Model file for the job. Use its own axes, mm. A direction names the side the tool comes from. Give positions to 0.01 mm unless a question says otherwise; leave off trailing zeros. Write each loop counter-clockwise with the first axis right and the second up, starting at its lowest first coordinate (ties: lowest second). Pieces come first, ordered by that corner, then holes. Notation, with made-up numbers: (51.25, -0.5) - (88.25, -0.5) arc R11 ccw to (88.25, 9.5) - close; hole circle Ø8 at (57, -17.5). An arc over 180 degrees is marked (long way). Use CSV: the item, a comma, the result in double quotes.
from build123d import *

# Parameters (mm, degrees)
BOSS_EXTRUDE1_DEPTH     = 1.5
BOSS_EXTRUDE2_DEPTH     = 280
SKETCH4_W               = 400
SKETCH4_H               = 42.385541564
BOSS_EXTRUDE3_DEPTH     = 2
CUT_EXTRUDE1_DEPTH      = 609.61485268
CUT_EXTRUDE1_DEPTH_BACK = 609.61485268
SKETCH8_R               = 4.39
SKETCH8_R_2             = 2.39
BOSS_EXTRUDE5_DEPTH     = 15
SKETCH10_R              = 3
CUT_EXTRUDE2_DEPTH      = 2
SKETCH15_W              = 15
SKETCH15_H              = 1.5
BOSS_EXTRUDE6_DEPTH     = 15
BOSS_EXTRUDE7_DEPTH     = 1.5
BOSS_EXTRUDE8_DEPTH     = 1.5
SKETCH20_R              = 2.415919743
SKETCH20_R_2            = 2
CUT_EXTRUDE5_DEPTH      = 1.5
SKETCH5_R               = 2
SKETCH5_R_2             = 10
CUT_EXTRUDE7_DEPTH      = 2
SKETCH21_W              = 300
SKETCH21_H              = 1.5
BOSS_EXTRUDE9_DEPTH     = 10
SKETCH22_W              = 300
SKETCH22_H              = 1.5
BOSS_EXTRUDE10_DEPTH    = 10
BOSS_EXTRUDE11_DEPTH    = 0.75
BOSS_EXTRUDE12_DEPTH    = 0.75
BOSS_EXTRUDE13_DEPTH    = 0.75
BOSS_EXTRUDE14_DEPTH    = 0.75
SKETCH27_W              = 200
SKETCH27_H              = 1.5
BOSS_EXTRUDE15_DEPTH    = 10
BOSS_EXTRUDE16_DEPTH    = 0.75
BOSS_EXTRUDE17_DEPTH    = 0.75
SKETCH30_R              = 24
SKETCH30_R_2            = 1.5
CUT_EXTRUDE8_DEPTH      = 2
SKETCH33_R              = 2
CUT_EXTRUDE9_DEPTH      = 2
SKETCH42_W              = 396
SKETCH42_H              = 39.39
CUT_EXTRUDE13_DEPTH     = 40


with BuildPart() as part:
    # Sketch1 → Boss-Extrude1 (new body)
    with BuildSketch(Plane(origin=(0, 0, 0), x_dir=(1, 0, 0), z_dir=(0, 1, 0))):
        Polygon((-200, 237.826300096), (200, 237.826300096), (200, -292.173699904), (150, -292.173699904), (150, -362.173699904), (-200, -362.173699904), align=None)
    extrude(amount=BOSS_EXTRUDE1_DEPTH)

    # Sketch2 → Boss-Extrude2 (add)
    with BuildSketch(Plane(origin=(0, 1.5, 0), x_dir=(1, 0, 0), z_dir=(0, 1, 0))):
        Polygon((-200, 237.826300096), (-200, -362.173699904), (150, -362.173699904), (150, -292.173699904), (200, -292.173699904), (200, 237.826300096), align=None)
        Polygon((-198, 235.826300096), (-198, -360.173699904), (148, -360.173699904), (148, -290.173699904), (198, -290.173699904), (198, 235.826300096), align=None, mode=Mode.SUBTRACT)
    extrude(amount=BOSS_EXTRUDE2_DEPTH)

    # Sketch4 → Boss-Extrude3 (add)
    with BuildSketch(Plane(origin=(0, 0, -237.826300096), x_dir=(-1, 0, 0), z_dir=(0, 0, -1))):
        with Locations((0, 213.483316708)):
            Rectangle(SKETCH4_W, SKETCH4_H)
    extrude(amount=-BOSS_EXTRUDE3_DEPTH)

    # Sketch3 → Cut-Extrude1 (cut, two sides: drawn at the far end of the back side and taken through both)
    with BuildSketch(Plane.ZY.offset(200).offset(-CUT_EXTRUDE1_DEPTH_BACK)):
        Polygon((362.173699904, 121.117558148), (228.195222706, 281.5), (362.173699904, 281.5), align=None)
    extrude(amount=CUT_EXTRUDE1_DEPTH + CUT_EXTRUDE1_DEPTH_BACK, mode=Mode.SUBTRACT)

    # Sketch8 → Boss-Extrude5 (add)
    # profile 1 of 2: a face of its own
    with BuildSketch(Plane(origin=(-198, 0, 0), x_dir=(0, 0, -1), z_dir=(1, 0, 0))):
        with Locations((-265.673697326, 172.19919718)):
            Circle(SKETCH8_R)
        with Locations((-265.673697326, 172.19919718)):
            Circle(SKETCH8_R_2, mode=Mode.SUBTRACT)
    # profile 2 of 2: a face of its own
    with BuildSketch(Plane(origin=(-198, 0, 0), x_dir=(0, 0, -1), z_dir=(1, 0, 0))):
        with Locations((-265.173699904, 16.5)):
            Circle(SKETCH8_R)
        with Locations((-265.173699904, 16.5)):
            Circle(SKETCH8_R_2, mode=Mode.SUBTRACT)
    extrude(amount=BOSS_EXTRUDE5_DEPTH)

    # Sketch10 → Cut-Extrude2 (cut)
    with BuildSketch(Plane.ZY.offset(-148)):
        with BuildLine():
            Line((333.923699904, 90.5), (319.923699904, 90.5))
            Line((319.923699904, 90.5), (319.923699904, 87.5))
            Line((319.923699904, 87.5), (315.673699904, 87.5))
            ThreePointArc((315.673699904, 87.5), (304.673699904, 76.5), (315.673699904, 65.5))
            Line((315.673699904, 65.5), (338.173699904, 65.5))
            ThreePointArc((338.173699904, 65.5), (349.173699904, 76.5), (338.173699904, 87.5))
            Line((338.173699904, 87.5), (333.923699904, 87.5))
            Line((333.923699904, 87.5), (333.923699904, 90.5))
        make_face()
        with Locations((300.973699904, 103.45)):
            Circle(SKETCH10_R)
        with Locations((352.873699904, 103.45)):
            Circle(SKETCH10_R)
        with Locations((300.973699904, 49.55)):
            Circle(SKETCH10_R)
        with Locations((352.873699904, 49.55)):
            Circle(SKETCH10_R)
    extrude(amount=-CUT_EXTRUDE2_DEPTH, mode=Mode.SUBTRACT)

    # Sketch15 → Boss-Extrude6 (add)
    with BuildSketch(Plane.ZY.offset(-198)):
        with Locations((-216.326300096, 251.386283415)):
            Rectangle(SKETCH15_W, SKETCH15_H)
        with Locations((203.673699904, 251.386283415)):
            Rectangle(SKETCH15_W, SKETCH15_H)
    extrude(amount=BOSS_EXTRUDE6_DEPTH)

    # Sketch17 → Boss-Extrude7 (add)
    with BuildSketch(Plane.XY.offset(-208.826300096)):
        Polygon((198, 250.636283415), (198, 235.636283415), (183, 250.636283415), align=None)
    extrude(amount=-BOSS_EXTRUDE7_DEPTH)

    # Sketch18 → Boss-Extrude8 (add)
    with BuildSketch(Plane.XY.offset(196.173699904)):
        Polygon((198, 250.636283415), (198, 235.636283415), (183, 250.636283415), align=None)
    extrude(amount=BOSS_EXTRUDE8_DEPTH)

    # Sketch20 → Cut-Extrude5 (cut)
    with BuildSketch(Plane(origin=(0, 252.136283415, 0), x_dir=(1, 0, 0), z_dir=(0, 1, 0))):
        with Locations(Location((190.5, 216.326300096, 0), (0, 0, 270))):
            Circle(SKETCH20_R)
        with Locations(Location((190.5, -203.673699904, 0), (0, 0, 270))):
            Circle(SKETCH20_R_2)
    extrude(amount=-CUT_EXTRUDE5_DEPTH, mode=Mode.SUBTRACT)

    # Sketch5 → Cut-Extrude7 (cut)
    with BuildSketch(Plane.ZY.offset(200)):
        with Locations((-115.826300096, 247.120648807)):
            Circle(SKETCH5_R)
        with Locations((-116.326300096, 223.125857706)):
            Circle(SKETCH5_R)
        with Locations((-91.826300096, 223.120648807)):
            Circle(SKETCH5_R)
        with Locations((-91.826300096, 247.120648807)):
            Circle(SKETCH5_R)
        with Locations((-103.826300096, 235.120648807)):
            Circle(SKETCH5_R_2)
        with Locations((-55.826300096, 247.120648807)):
            Circle(SKETCH5_R)
        with Locations((-56.326300096, 223.125857706)):
            Circle(SKETCH5_R)
        with Locations((-31.826300096, 223.120648807)):
            Circle(SKETCH5_R)
        with Locations((-31.826300096, 247.120648807)):
            Circle(SKETCH5_R)
        with Locations((-43.826300096, 235.120648807)):
            Circle(SKETCH5_R_2)
        with Locations((4.173699904, 247.120648807)):
            Circle(SKETCH5_R)
        with Locations((3.673699904, 223.125857706)):
            Circle(SKETCH5_R)
        with Locations((28.173699904, 223.120648807)):
            Circle(SKETCH5_R)
        with Locations((28.173699904, 247.120648807)):
            Circle(SKETCH5_R)
        with Locations((16.173699904, 235.120648807)):
            Circle(SKETCH5_R_2)
        with Locations((64.173699904, 247.120648807)):
            Circle(SKETCH5_R)
        with Locations((63.673699904, 223.125857706)):
            Circle(SKETCH5_R)
        with Locations((88.173699904, 223.120648807)):
            Circle(SKETCH5_R)
        with Locations((88.173699904, 247.120648807)):
            Circle(SKETCH5_R)
        with Locations((76.173699904, 235.120648807)):
            Circle(SKETCH5_R_2)
    extrude(amount=-CUT_EXTRUDE7_DEPTH, mode=Mode.SUBTRACT)

    # Sketch21 → Boss-Extrude9 (add)
    with BuildSketch(Plane(origin=(0, 0, -237.826300096), x_dir=(-1, 0, 0), z_dir=(0, 0, -1))):
        with Locations((0, 270.75)):
            Rectangle(SKETCH21_W, SKETCH21_H)
    extrude(amount=BOSS_EXTRUDE9_DEPTH)

    # Sketch22 → Boss-Extrude10 (add)
    with BuildSketch(Plane.ZY.offset(200)):
        with Locations((-7.826300096, 270.75)):
            Rectangle(SKETCH22_W, SKETCH22_H)
    boss_extrude10 = extrude(amount=BOSS_EXTRUDE10_DEPTH)

    # Sketch23 → Boss-Extrude11 (add, symmetric)
    with BuildSketch(Plane(origin=(0, 0, -77.826300096), x_dir=(-1, 0, 0), z_dir=(0, 0, -1))):
        Polygon((210, 270), (200, 270), (200, 260), align=None)
    boss_extrude11 = extrude(amount=BOSS_EXTRUDE11_DEPTH, both=True)

    # Sketch24 → Boss-Extrude12 (add, symmetric)
    with BuildSketch(Plane.XY.offset(52.173699904)):
        Polygon((-210, 270), (-200, 260), (-200, 270), align=None)
    boss_extrude12 = extrude(amount=BOSS_EXTRUDE12_DEPTH, both=True)

    # Sketch25 → Boss-Extrude13 (add, symmetric)
    with BuildSketch(Plane(origin=(100, 0, 0), x_dir=(0, 0, -1), z_dir=(1, 0, 0))):
        Polygon((247.826300096, 270), (237.826300096, 270), (237.826300096, 260), align=None)
    extrude(amount=BOSS_EXTRUDE13_DEPTH, both=True)

    # Sketch26 → Boss-Extrude14 (add, symmetric)
    with BuildSketch(Plane.ZY.offset(100)):
        Polygon((-247.826300096, 270), (-237.826300096, 260), (-237.826300096, 270), align=None)
    extrude(amount=BOSS_EXTRUDE14_DEPTH, both=True)

    # Mirror1: Boss-Extrude10, Boss-Extrude11, Boss-Extrude12 across plane
    add(boss_extrude10.mirror(Plane(origin=(0, 0, 0), x_dir=(0, 0, 1), z_dir=(1, 0, 0))))
    add(boss_extrude11.mirror(Plane(origin=(0, 0, 0), x_dir=(0, 0, 1), z_dir=(1, 0, 0))))
    add(boss_extrude12.mirror(Plane(origin=(0, 0, 0), x_dir=(0, 0, 1), z_dir=(1, 0, 0))))

    # Sketch27 → Boss-Extrude15 (add)
    with BuildSketch(Plane.XY.offset(362.173699904)):
        with Locations((-25, 110.367558148)):
            Rectangle(SKETCH27_W, SKETCH27_H)
    extrude(amount=BOSS_EXTRUDE15_DEPTH)

    # Sketch28 → Boss-Extrude16 (add, symmetric)
    with BuildSketch(Plane.ZY.offset(95)):
        Polygon((372.173699904, 109.617558148), (362.173699904, 109.617558148), (362.173699904, 99.617558148), align=None)
    extrude(amount=BOSS_EXTRUDE16_DEPTH, both=True)

    # Sketch29 → Boss-Extrude17 (add, symmetric)
    with BuildSketch(Plane(origin=(45, 0, 0), x_dir=(0, 0, -1), z_dir=(1, 0, 0))):
        Polygon((-372.173699904, 109.617558148), (-362.173699904, 99.617558148), (-362.173699904, 109.617558148), align=None)
    extrude(amount=BOSS_EXTRUDE17_DEPTH, both=True)

    # Sketch30 → Cut-Extrude8 (cut)
    with BuildSketch(Plane(origin=(200, 0, 0), x_dir=(0, 0, -1), z_dir=(1, 0, 0))):
        with Locations((-258.673699904, 160)):
            Circle(SKETCH30_R)
        with Locations((-284.673699904, 150)):
            Circle(SKETCH30_R_2)
        with Locations((-232.673699904, 150)):
            Circle(SKETCH30_R_2)
    extrude(amount=-CUT_EXTRUDE8_DEPTH, mode=Mode.SUBTRACT)

    # Sketch33 → Cut-Extrude9 (cut)
    with BuildSketch(Plane.ZY.offset(200)):
        with Locations((-180.626300096, 147.77)):
            Circle(SKETCH33_R)
        with Locations((-180.626300096, 28.39)):
            Circle(SKETCH33_R)
        with Locations((-8.926300096, 147.77)):
            Circle(SKETCH33_R)
        with Locations((-8.926300096, 28.39)):
            Circle(SKETCH33_R)
        with Locations((162.773699904, 147.77)):
            Circle(SKETCH33_R)
        with Locations((162.773699904, 28.39)):
            Circle(SKETCH33_R)
    extrude(amount=-CUT_EXTRUDE9_DEPTH, mode=Mode.SUBTRACT)

    # Sketch42 → Cut-Extrude13 (cut)
    with BuildSketch(Plane.XY.offset(-235.826300096)):
        with Locations((0, 213.485)):
            Rectangle(SKETCH42_W, SKETCH42_H)
    extrude(amount=-CUT_EXTRUDE13_DEPTH, mode=Mode.SUBTRACT)


solid = part.part
(1) Wall check: probe 1 along Z at (x, y) = (-123, 69.5); probe 2 along X at (y, z) = (215, -87); probe 3 along Z at (x, y) = (153.5, 17). Give the ranges that are in metal, low to high. Write a range as [from, to].
Checked values:
probe 1,"z = [-237.83, -235.83], [360.17, 362.17]"
probe 2,"x = [-200, -198], [198, 200]"
probe 3,"z = [-237.83, -235.83], [290.17, 292.17]"
(2) Saw through at B-B, the plane z = -106.5. List the corners of the cut face in (x, y), then the cut area to 3 significant figures.
Checked values:
outline,"(-210, 270) - (-200, 270) - (-200, 244.76) - (-198, 244.76) - (-198, 281.5) - (-200, 281.5) - (-200, 271.5) - (-210, 271.5) - close; (-200, 0) - (200, 0) - (200, 270) - (210, 270) - (210, 271.5) - (200, 271.5) - (200, 281.5) - (198, 281.5) - (198, 1.5) - (-198, 1.5) - (-198, 225.48) - (-200, 225.48) - close"
area,"1,710 mm^2"
(3) Pull direction Y, two halves, no side cores. Call faces 4 (the face through (192.3, 252.136, 205.2)), 5 (the face through (190.605, 243.031, -209.566)), 6 (the face through (3, 257, -235.826)): released by +Y, released by -Y, zero draft, split by the parting line, or undercut.
Checked values:
face 4,"released by +Y"
face 5,"undercut"
face 6,"zero draft"
(4) 3-axis set-ups, long thin cutter, end or side, ignore diameter. For faces 1 (the face through (148, 103, 326)), 2 (the face through (150, 101, 328)), 3 (the face through (-199.01, 231.29, -94.59)): which of +Z, -Z, +X, -X, +Y, -Y reach the whole face in a straight line?
Checked values:
face 1,"+Y"
face 2,"+Z, +X, +Y, -Y"
face 3,"-X"
(5) Saw through at C-C, the plane y = 76.5. List the corners of the cut face in (x, z).
Checked values:
outline,"(-200, -237.83) - (200, -237.83) - (200, 292.17) - (150, 292.17) - (150, 304.67) - (148, 304.67) - (148, 290.17) - (198, 290.17) - (198, -235.83) - (-198, -235.83) - (-198, 360.17) - (148, 360.17) - (148, 349.17) - (150, 349.17) - (150, 362.17) - (-200, 362.17) - close"
(6) Saw through at D-D, the plane z = 40.5. List the corners of the cut face in (x, y), then the cut area to 3 significant figures.
Checked values:
outline,"(-210, 270) - (-200, 270) - (-200, 0) - (200, 0) - (200, 270) - (210, 270) - (210, 271.5) - (200, 271.5) - (200, 281.5) - (198, 281.5) - (198, 1.5) - (-198, 1.5) - (-198, 281.5) - (-200, 281.5) - (-200, 271.5) - (-210, 271.5) - close"
area,"1,750 mm^2"
(7) Flat gauge pins, fed straight in: P1, Ø3, axis at y = 119.5, z = 123, coming from the +X side; P2, Ø4, axis at x = 75.5, y = 100.5, coming from the +Z side; P3, Ø1.6, axis at y = 271, z = -242.5, coming from the +X side. Where does each tip first touch, or does it go through?
Checked values:
P1,"stops at x = 200"
P2,"stops at z = 362.17"
P3,"stops at x = 150"
(8) Saw through at A-A, the plane x = 132. List the corners of the cut face in (y, z), then the cut area to 3 significant figures.
Checked values:
outline,"(0, -237.83) - (193.79, -237.83) - (193.79, -235.83) - (1.5, -235.83) - (1.5, 360.17) - (123.51, 360.17) - (121.12, 362.17) - (0, 362.17) - close; (233.18, -237.83) - (270, -237.83) - (270, -247.83) - (271.5, -247.83) - (271.5, -237.83) - (281.5, -237.83) - (281.5, -235.83) - (233.18, -235.83) - close"
area,"1,640 mm^2"
